Design review of the part built by this model. Coordinates are the model's own, in mm. A direction names the side the tool comes from. Give positions to 0.01 mm unless a question says otherwise; leave off trailing zeros. Loops run counter-clockwise (first coordinate to the right, second up) from the corner with the lowest first, then second, coordinate; pieces in that order, holes last. Notation, with made-up numbers: M 28.5,45 L 34.5,45 A23 cw 34.5,66 Z; hole C 3,1 d2. An arc over 180 degrees is marked long. Use a Markdown table: item, result. Add a question column.
(1) For faces 1 (the face through (3.969, -14, 5)), 2 (the face through (-3.969, -14, 5)), 3 (the face through (-11.107, 0.356, 5.892)), 4 (the face through (-3.969, 14, 5)), list the 3-axis set-ups (+Z, -Z, +X, -X, +Y, -Y) from which the entire face can be reached by the end or side of a thin tool; tool diameter is ignored.
(2) For probe 1 along Y at (x, z) = (0, 4.5); probe 2 along Y at (x, z) = (0, 1.2) (3 decimals); probe 3 along Z at (x, y) = (-6, 8.5), list the stretches that pass through material, from the lowest coordinate up.
(3) Add section D-D, the plane x = -10. Give the boundary of the cut face in (y, z), then the cut area to 3 significant figures.
(4) Add section A-A, the plane x = 0. State how many separate pieces and enclosed holes the cut face has, then the cut area to 3 significant figures.
(5) Draft analysis for pull direction Y (two halves, no side actions). For faces 5 (the face through (5.7, -13.1, 5.1)), 6 (the face through (-9, 4, 1.588)), 7 (the face through (-11, 3, 10.319)), state which applies: pulls with the +Y half, pulls with the -Y half, needs draft (parallel to the pull), parting line crosses it, or undercut.
(6) Add section B-B, the plane z = 2.5. Give the boundary of the cut face in (x, y) (1 decimal).
(7) Insertion check: pin 1 Ø1 at (x, z) = (-4, 9) entering from +Y; pin 2 Ø1.5 at (y, z) = (-14, 5) entering from +X; pin 3 Ø1.1 at (y, z) = (14.5, 3) entering from +X; pin 4 Ø2.5 at (x, y) = (0, -15.08) entering from +Z. Each pin has a flat end and moves straight along its axis. Give the tip position at first contact, or say it passes through.
(8) Add section C-C, the plane y = 0. Give the boundary of the cut face in (x, z) (1 decimal), then the cut area to 3 significant figures.
```python
from build123d import *

# Parameters (mm, degrees)
F0_R     = 2.2479
F0_R_2   = 9.525
F1_DEPTH = 1.5875
F2_R     = 2.2479
F2_R_2   = 11.1125
F3_DEPTH = 8.73125
F5_DEPTH = 10.31875


with BuildPart() as f1:
    # F0 (on Top) → F1 (new body)
    with BuildSketch(Plane.XY):
        with BuildLine():
            Line((3.96875, -15.08125), (3.96875, -13.725221))
            ThreePointArc((3.96875, -13.725221), (14.2875, 0), (3.96875, 13.725221))
            Line((3.96875, 13.725221), (3.96875, 15.08125))
            ThreePointArc((3.96875, 15.08125), (0, 19.05), (-3.96875, 15.08125))
            Line((-3.96875, 15.08125), (-3.96875, 13.725221))
            ThreePointArc((-3.96875, 13.725221), (-14.2875, 0), (-3.96875, -13.725221))
            Line((-3.96875, -13.725221), (-3.96875, -15.08125))
            ThreePointArc((-3.96875, -15.08125), (0, -19.05), (3.96875, -15.08125))
        make_face()
        with Locations((0, -15.08125)):
            Circle(F0_R, mode=Mode.SUBTRACT)
        Circle(F0_R_2, mode=Mode.SUBTRACT)
        with Locations((0, 15.08125)):
            Circle(F0_R, mode=Mode.SUBTRACT)
    extrude(amount=F1_DEPTH)

    # F2 (on face) → F3 (join)
    with BuildSketch(Plane.XY.offset(1.5875)):
        with BuildLine():
            ThreePointArc((-3.96875, 13.725221), (-14.2875, 0), (-3.96875, -13.725221))
            Line((-3.96875, -13.725221), (-3.96875, -15.08125))
            ThreePointArc((-3.96875, -15.08125), (0, -19.05), (3.96875, -15.08125))
            Line((3.96875, -15.08125), (3.96875, -13.725221))
            ThreePointArc((3.96875, -13.725221), (14.2875, 0), (3.96875, 13.725221))
            Line((3.96875, 13.725221), (3.96875, 15.08125))
            ThreePointArc((3.96875, 15.08125), (0, 19.05), (-3.96875, 15.08125))
            Line((-3.96875, 15.08125), (-3.96875, 13.725221))
        make_face()
        with Locations((0, -15.08125)):
            Circle(F2_R, mode=Mode.SUBTRACT)
        Circle(F2_R_2, mode=Mode.SUBTRACT)
        with Locations((0, 15.08125)):
            Circle(F2_R, mode=Mode.SUBTRACT)
    extrude(amount=F3_DEPTH)

    # F4 (on face) → F5 (cut, through all)
    with BuildSketch(Plane.XY.offset(10.31875)):
        Polygon((7.304354, 0), (7.304354, -14.2875), (14.2875, -14.2875), (14.2875, 14.2875), (7.304354, 14.2875), align=None)
    extrude(amount=-F5_DEPTH, mode=Mode.SUBTRACT)


solid = f1.part
```
Established:
| question | item | result |
|---|---|---|
| 1 | face 1 | +Z, -Z, +X, -Y |
| 1 | face 2 | +Z, -Z, -X, -Y |
| 1 | face 3 | +Z |
| 1 | face 4 | +Z, -Z, -X, +Y |
| 2 | probe 1 | -19.05 to -17.33, -12.83 to -11.11, 11.11 to 12.83, 17.33 to 19.05 |
| 2 | probe 2 | -19.05 to -17.329, -12.833 to -9.525, 9.525 to 12.833, 17.329 to 19.05 |
| 2 | probe 3 | 0 to 1.59 |
| 3 | outline | M -10.2,0 L 10.2,0 L 10.2,10.32 L 4.85,10.32 L 4.85,1.59 L -4.85,1.59 L -4.85,10.32 L -10.2,10.32 Z |
| 3 | area | 126 mm^2 |
| 4 | separate pieces | 4 |
| 4 | enclosed holes | 0 |
| 4 | area | 76.1 mm^2 |
| 5 | face 5 | pulls with the -Y half |
| 5 | face 6 | undercut |
| 5 | face 7 | needs draft |
| 6 | outline | M -4,-15.1 A4 ccw 4,-15.1 L 4,-13.7 A14.3 ccw 7.3,-12.3 L 7.3,-8.4 A11.1 cw long 7.3,8.4 L 7.3,12.3 A14.3 ccw 4,13.7 L 4,15.1 A4 ccw -4,15.1 L -4,13.7 A14.3 ccw -4,-13.7 Z; hole C 0,-15.1 d4.5; hole C 0,15.1 d4.5 |
| 7 | pin 1 | y = 16.95 |
| 7 | pin 2 | x = 5.35 |
| 7 | pin 3 | x = 3.97 |
| 7 | pin 4 | through |
| 8 | outline | M -14.3,0 L -9.5,0 L -9.5,1.6 L -11.1,1.6 L -11.1,10.3 L -14.3,10.3 Z |
| 8 | area | 35.3 mm^2 |
